The model under review builds one solid part; all positions refer to its coordinate system, in mm. Face numbers are marked on the shaded views. A direction names the side the tool comes from. Round coordinates to 2 decimals unless told otherwise and drop trailing zeros. Loops run counter-clockwise (first coordinate to the right, second up) from the corner with the lowest first, then second, coordinate; pieces in that order, holes last. Notation, with made-up numbers: (1.5, -33.75) -> (40.5, -33.75) arc R30 ccw to (40.5, -5.75) -> close; hole circle Ø10 at (40.5, 50.5). An arc over 180 degrees is marked (long way). Use a Markdown table: item, result. Add a question column.
1) For the marked faces 1 and 2, list the 3-axis set-ups (+Z, -Z, +X, -X, +Y, -Y) from which the entire face can be reached by the end or side of a thin tool; tool diameter is ignored.
2) Consider section D-D on x = 33.5. Give the boundary of the cut face in (y, z), plus the area to 3 significant figures.
3) Consider section A-A on z = 17.5. Give the boundary of the cut face in (x, y), plus the area to 3 significant figures.
4) Consider section B-B on y = -6.5. Give the boundary of the cut face in (x, z), plus the area to 3 significant figures.
5) Wall thickness on probe 1 along Z at (x, y) = (22, 0.5); probe 2 along X at (y, z) = (23, 54); probe 3 along Z at (x, y) = (-27.5, -13.5): over which ranges is each line inside the solid? List them lowest first.
6) Insertion check: pin 1 (7.5 mm diameter, centred on x = -37.5, z = 19, fed in from +Y); pin 2 (3 mm diameter, centred on x = -21.5, y = -8.5, fed in from +Z); pin 3 (0.5 mm diameter, centred on x = 3.5, y = 28, fed in from +Z); pin 4 (8 mm diameter, centred on x = -26.5, z = 39, fed in from -Y). Each pin has a flat end and moves straight along its axis. Give the tip position at first contact, or say it passes through.
7) Consider section C-C on x = -22. Give the boundary of the cut face in (y, z).
8) Mouldability with a two-part tool opening along Y and no side actions: class the marked faces 3, 4 and 5 as released by +Y, released by -Y, zero draft, split by the parting line, or undercut.
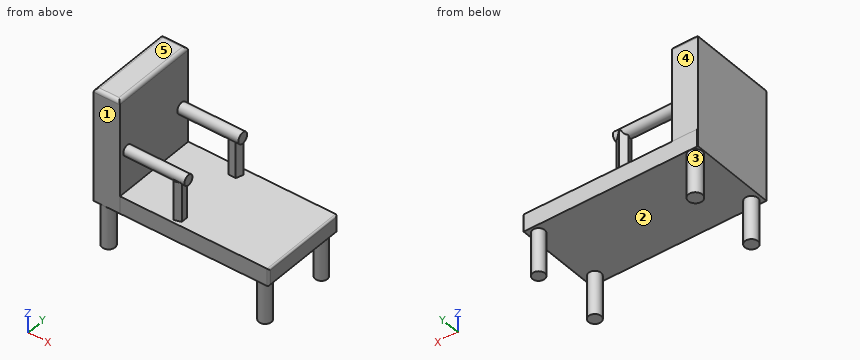
from build123d import *

# Parameters (mm, degrees)
F0_W     = 100
F0_H     = 50
F1_DEPTH = 10
F2_R     = 3.601713
F2_R_2   = 3.485572
F2_R_3   = 3.723077
F2_R_4   = 4
F3_DEPTH = 25
F4_W     = 15
F4_H     = 50
F5_DEPTH = 65
F6_R     = 2.976027
F6_R_2   = 3.210208
F7_DEPTH = 35
F9_DEPTH = 22.4
F10_R    = 2
F11_R    = 1


with BuildPart() as f1:
    # F0 (on Top) → F1 (new body)
    with BuildSketch(Plane.XY):
        with Locations((7.828464, 4.295976)):
            Rectangle(F0_W, F0_H)
    extrude(amount=F1_DEPTH)

    # F2 (on face) → F3 (join)
    with BuildSketch(Plane(origin=(0, 0, 0), x_dir=(1, 0, 0), z_dir=(0, 0, -1))):
        with Locations((51.622987, 15.514113)):
            Circle(F2_R)
        with Locations((52.530244, -24.405243)):
            Circle(F2_R_2)
        with Locations((-37.106857, 16.784275)):
            Circle(F2_R_3)
        with Locations((-37.832662, -25.13105)):
            Circle(F2_R_4)
    extrude(amount=F3_DEPTH)

    # F4 (on Top) → F5 (join)
    with BuildSketch(Plane.XY):
        with Locations((-35.050407, 4.223788)):
            Rectangle(F4_W, F4_H)
    extrude(amount=F5_DEPTH)

    # F6 (on face) → F7 (join)
    with BuildSketch(Plane.YZ.offset(-27.550407)):
        with Locations((-15.28226, 33.31653)):
            Circle(F6_R)
        with Locations((24.455646, 32.590725)):
            Circle(F6_R_2)
    extrude(amount=F7_DEPTH)

    # F8 (on face) → F9 (join)
    with BuildSketch(Plane.XY.offset(10)):
        Polygon((5.741771, -17.913366), (5.741771, -13.958396), (1.980372, -12.736244), (-0.344301, -15.935881), (1.980372, -19.135518), align=None)
        Polygon((1.273584, 21.806058), (5.492217, 21.806058), (6.795846, 25.818216), (3.3829, 28.297866), (-0.030045, 25.818216), align=None)
    extrude(amount=F9_DEPTH)

    # F10
    f10_edges = [f1.edges().sort_by_distance(p)[0] for p in [
        (-42.550407, 4.223788, 65),
        (-35.050407, -20.776212, 65),
        (-27.550407, 4.223788, 65),
        (-35.050407, 29.223788, 65),
    ]]
    fillet(f10_edges, radius=F10_R)

    # F11
    f11_edges = [f1.edges().sort_by_distance(p)[0] for p in [
        (57.828464, -20.704024, 5),
        (57.828464, 29.295976, 5),
        (57.828464, 4.295976, 0),
        (57.828464, 4.295976, 10),
    ]]
    fillet(f11_edges, radius=F11_R)


solid = f1.part
Result set:
| question | item | result |
|---|---|---|
| 1 | face 1 | +Z, -Z, +X, -X, -Y |
| 1 | face 2 | -Z |
| 2 | outline | (-20.7, 0) -> (29.3, 0) -> (29.3, 10) -> (-20.7, 10) -> close |
| 2 | area | 500 mm2 |
| 3 | outline | (-42.55, -20.78) -> (-27.55, -20.78) -> (-27.55, 29.22) -> (-42.55, 29.22) -> close; (-0.34, -15.94) -> (1.98, -19.14) -> (5.74, -17.91) -> (5.74, -13.96) -> (1.98, -12.74) -> close; (-0.03, 25.82) -> (1.27, 21.81) -> (5.49, 21.81) -> (6.8, 25.82) -> (3.38, 28.3) -> close |
| 3 | area | 808 mm2 |
| 4 | outline | (-42.55, 0) -> (56.83, 0) arc R1 ccw to (57.83, 1) -> (57.83, 9) arc R1 ccw to (56.83, 10) -> (-27.55, 10) -> (-27.55, 63) arc R2 ccw to (-29.55, 65) -> (-40.55, 65) arc R2 ccw to (-42.55, 63) -> close |
| 4 | area | 1,830 mm2 |
| 5 | probe 1 | 0 to 10 |
| 5 | probe 2 | -42.55 to -27.55 |
| 5 | probe 3 | 0 to 10, 30.93 to 35.7 |
| 6 | pin 1 | y = 29.22 |
| 6 | pin 2 | z = 10 |
| 6 | pin 3 | z = 32.4 |
| 6 | pin 4 | y = -20.78 |
| 7 | outline | (-20.7, 0) -> (29.3, 0) -> (29.3, 10) -> (-20.7, 10) -> close; circle Ø5.95 at (-15.28, 33.32); circle Ø6.42 at (24.46, 32.59) |
| 8 | face 3 | undercut |
| 8 | face 4 | released by +Y |
| 8 | face 5 | zero draft |
